```python
from build123d import *

# Parameters (mm, degrees)
SKETCH1_R           = 78.613
BOSS_EXTRUDE1_DEPTH = 228.6
SKETCH2_W           = 3.175
SKETCH2_H           = 194.31
CUT_EXTRUDE1_DEPTH  = 203.2
SKETCH5_W           = 194.31
SKETCH5_H           = 3.175
CUT_EXTRUDE2_DEPTH  = 203.2


with BuildPart() as part:
    # Sketch1 → Boss-Extrude1 (new body)
    with BuildSketch(Plane.XY):
        Polygon((77.066602343, -42.148481212), (84.297794001, 24.690840238), (42.148481212, 77.066602343), (-24.690840238, 84.297794001), (-77.066602343, 42.148481212), (-84.297794001, -24.690840238), (-42.148481212, -77.066602343), (24.690840238, -84.297794001), align=None)
        Circle(SKETCH1_R, mode=Mode.SUBTRACT)
    extrude(amount=BOSS_EXTRUDE1_DEPTH)

    # Sketch2 → Cut-Extrude1 (cut)
    with BuildSketch(Plane(origin=(8.728820487, 80.682198172, 0), x_dir=(0.99419859, -0.107560047, 0), z_dir=(0.107560047, 0.99419859, 0))):
        with Locations((0, -122.555)):
            Rectangle(SKETCH2_W, SKETCH2_H)
    extrude(amount=-CUT_EXTRUDE1_DEPTH, mode=Mode.SUBTRACT)

    # Sketch5 → Cut-Extrude2 (cut)
    with BuildSketch(Plane(origin=(-80.682198172, 8.728820487, 0), x_dir=(0, 0, 1), z_dir=(-0.99419859, 0.107560047, 0))):
        with Locations((122.555, 0)):
            Rectangle(SKETCH5_W, SKETCH5_H)
    extrude(amount=-CUT_EXTRUDE2_DEPTH, mode=Mode.SUBTRACT)


solid = part.part
```
Verification items for the finished model (mm, model axes). Coordinates: 2 decimals unless noted, no trailing zeros. Loops run counter-clockwise (first coordinate to the right, second up) from the corner with the lowest first, then second, coordinate; pieces in that order, holes last. Notation, with made-up numbers: (-29.5, 71.25) -> (15.5, 71.25) arc R29 cw to (15.5, 102.25) -> close; hole circle Ø11 at (-1.5, 30.5). An arc over 180 degrees is marked (long way). Answer in a Markdown table with one row per item. Add a question column.
1. Section check A-A, the plane z = 136.5. Enter the section's corners in (x, y).
2. Material ranges on probe 1 along X at (y, z) = (-5.5, 105); probe 2 along Y at (x, z) = (30.5, 123.5); probe 3 along Y at (x, z) = (-32.5, 126), recorded low to high. Write a range as [from, to].
3. Section check C-C, the plane y = 54. Enter the section's corners in (x, z).
4. Draft check along Y on faces 1 (the face through (-69, 38, 0)), 2 (the face through (63.52, 50.51, 112.7)), 3 (the face through (50.51, -63.52, 112.7)), 4 (the face through (-17.042, -76.744, 112.7)). Enter one of: +Y half, -Y half, draft (parallel to the pull), parting line (faces both ways), or undercut.
5. Depth check by flat-ended pin: P1, Ø10, axis at x = 60, z = 100.5, coming from the +Y side; P2, Ø2, axis at y = 57.5, z = 170.5, coming from the -X side; P3, Ø5, axis at x = 58, z = 68.5, coming from the +Y side. Enter the tip coordinate at first touch or a pass-through.
6. Section check B-B, the plane x = 73. Enter the section's corners in (y, z).
Derived:
| question | item | result |
|---|---|---|
| 1 | outline | (-84.3, -24.69) -> (-42.15, -77.07) -> (-10.31, -80.51) -> (-10.03, -77.97) arc R78.61 cw to (-78.31, 6.88) -> (-80.85, 7.15) -> close; (-80.51, 10.31) -> (-77.97, 10.03) arc R78.61 cw to (6.88, 78.31) -> (7.15, 80.85) -> (-24.69, 84.3) -> (-77.07, 42.15) -> close; (-7.15, -80.85) -> (24.69, -84.3) -> (77.07, -42.15) -> (80.51, -10.31) -> (77.97, -10.03) arc R78.61 cw to (-6.88, -78.31) -> close; (10.03, 77.97) arc R78.61 cw to (78.31, -6.88) -> (80.85, -7.15) -> (84.3, 24.69) -> (42.15, 77.07) -> (10.31, 80.51) -> close |
| 2 | probe 1 | x = [-82.22, -78.42], [78.42, 81.03] |
| 2 | probe 2 | y = [-79.62, -72.46], [72.46, 78.33] |
| 2 | probe 3 | y = [-78.11, -71.58], [71.58, 78.01] |
| 3 | outline | (-62.34, 0) -> (-57.13, 0) -> (-57.13, 228.6) -> (-62.34, 228.6) -> close; (57.13, 0) -> (60.71, 0) -> (60.71, 228.6) -> (57.13, 228.6) -> close |
| 4 | face 1 | draft |
| 4 | face 2 | +Y half |
| 4 | face 3 | -Y half |
| 4 | face 4 | undercut |
| 5 | P1 | stops at y = 61.1 |
| 5 | P2 | stops at x = -59.23 |
| 5 | P3 | stops at y = 60.48 |
| 6 | outline | (-45.42, 0) -> (-29.17, 0) -> (-29.17, 228.6) -> (-45.42, 228.6) -> close; (29.17, 0) -> (38.73, 0) -> (38.73, 228.6) -> (29.17, 228.6) -> close |
